Geometry: final body of the model. Coordinates: model frame, mm. Face numbers are marked on the shaded views. A direction names the side the tool comes from. Coordinates: 2 decimals unless noted, no trailing zeros. Loops run counter-clockwise (first coordinate to the right, second up) from the corner with the lowest first, then second, coordinate; pieces in that order, holes last. Notation, with made-up numbers: (-12, -18.5) -> (46, -18.5) arc R15 cw to (46, -0.5) -> close; hole circle Ø11 at (8, -2). An arc over 180 degrees is marked (long way). One line per item, written item: value. Start each with the question number.
Item 1: Section query A-A on x = 0. Give the number of separate pieces and of enclosed holes in the cut face, then the cut area to 3 significant figures.
Item 2: Contact query for flat-ended pins moving along their axis: pin 1 Ø6 at (y, z) = (21.5, -11.5) entering from -X; pin 2 Ø6 at (x, z) = (0, 14.5) entering from -Y; pin 3 Ø3 at (x, z) = (-4.5, 12) entering from +Y. Output: stop coordinate, or through.
Item 3: Section query C-C on x = -13. Return loops of the section in (y, z).
Item 4: Ray query, probe 1 along Z at (x, y) = (0, 3.1); probe 2 along Z at (x, y) = (0, 4.6); probe 3 along Y at (x, z) = (16, 9). Return the intervals inside material, ascending. Write a range as from..to.
Item 5: Section query D-D on z = 14.5. Return loops of the section in (x, y).
Item 6: Mould query, pull axis Z, two halves, no side actions, for the marked faces 1, 2, 3 and 4. Classes: +Z half, -Z half, draft (parallel to the pull), parting line (faces both ways), or undercut.
Item 7: Set-up query: the marked faces 5, 6 and 7. Return all of +Z, -Z, +X, -X, +Y, -Y with unobstructed straight access to the full face (end or side cutting, diameter ignored); none if empty.
from build123d import *

# Parameters (mm, degrees)
F2_R     = 2.25
F3_DEPTH = 29.001
F4_R     = 3.75
F5_DEPTH = 4.1
F6_SIZE  = 0.6
F7_R     = 1


with BuildPart() as f1:
    # F0 (on Top) → F1 (revolve)
    with BuildSketch(Plane.XY):
        Polygon((5, 29), (5, 0), (20, 0), (20, 6), (9.5, 6), (9.5, 29), align=None)
    revolve(axis=Axis((0, 11.864793, 0), (0, 1, 0)))

    # F2 (on face) → F3 (cut, through all)
    with BuildSketch(Plane.XZ):
        with Locations((0, 14.5)):
            Circle(F2_R)
        with Locations((0, -14.5)):
            Circle(F2_R)
        with Locations((14.5, 0)):
            Circle(F2_R)
        with Locations((-14.5, 0)):
            Circle(F2_R)
    extrude(amount=-F3_DEPTH, mode=Mode.SUBTRACT)

    # F4 (on face) → F5 (cut)
    with BuildSketch(Plane.XZ):
        with Locations((0, 14.5)):
            Circle(F4_R)
        with Locations((14.5, 0)):
            Circle(F4_R)
        with Locations((0, -14.5)):
            Circle(F4_R)
        with Locations((-14.5, 0)):
            Circle(F4_R)
    extrude(amount=-F5_DEPTH, mode=Mode.SUBTRACT)

    # F6
    f6_edges = [f1.edges().sort_by_distance(p)[0] for p in [
        (5, 14.5, 0),
        (-5, 0, 0),
        (-5, 29, 0),
    ]]
    chamfer(f6_edges, length=F6_SIZE)

    # F7
    f7_edges = [f1.edges().sort_by_distance(p)[0] for p in [
        (-9.5, 6, 0),
    ]]
    fillet(f7_edges, radius=F7_R)


solid = f1.part
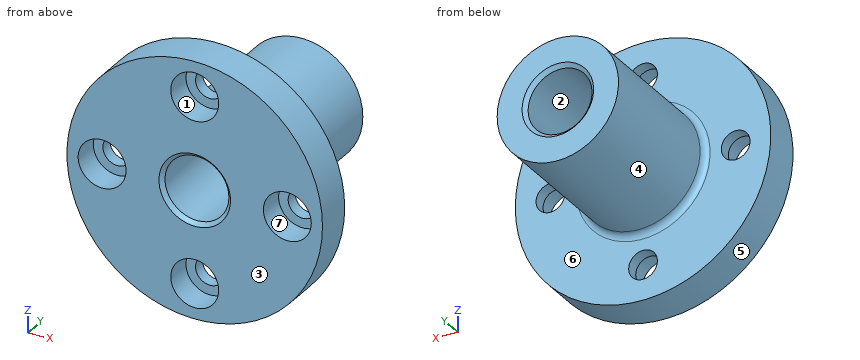
Reply:
1. separate pieces: 4
1. enclosed holes: 0
1. area: 308 mm²
2. pin 1: stops at x = -4.24
2. pin 2: stops at y = 4.1
2. pin 3: stops at y = 6
3. outline: (0, -15.2) -> (6, -15.2) -> (6, -1.68) -> (4.1, -1.68) -> (4.1, -3.44) -> (0, -3.44) -> close; (0, 3.44) -> (4.1, 3.44) -> (4.1, 1.68) -> (6, 1.68) -> (6, 15.2) -> (0, 15.2) -> close
4. probe 1: z = -20..-18.25, -10.75..-5, 5..10.75, 18.25..20
4. probe 2: z = -20..-16.75, -12.25..-5, 5..12.25, 16.75..20
4. probe 3: y = 0..6
5. outline: (-13.77, 0) -> (-3.75, 0) -> (-3.75, 4.1) -> (-2.25, 4.1) -> (-2.25, 6) -> (-13.77, 6) -> close; (2.25, 4.1) -> (3.75, 4.1) -> (3.75, 0) -> (13.77, 0) -> (13.77, 6) -> (2.25, 6) -> close
6. face 1: undercut
6. face 2: undercut
6. face 3: draft
6. face 4: parting line
7. face 5: +Y, -Y
7. face 6: +Y
7. face 7: -Y
